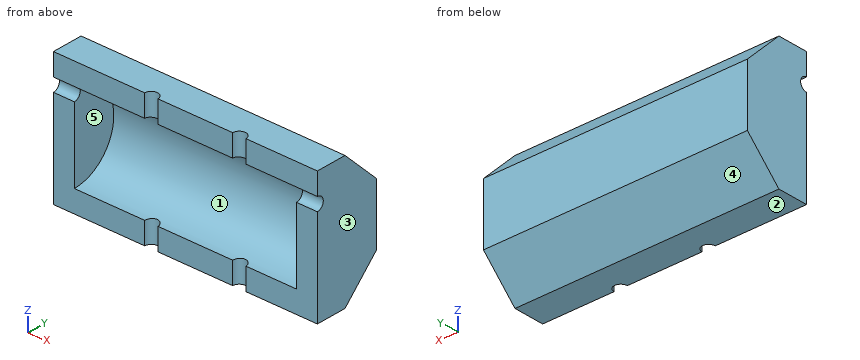
from build123d import *

# Parameters (mm, degrees)
F0_W          = 60
F0_H          = 30
F1_DEPTH      = 15
F3_W          = 50.5
F3_H          = 10
F5_R          = 1.5
F6_DEPTH      = 60.001
F7_R          = 1.5
F8_DEPTH      = 15.001
F8_DEPTH_BACK = 15.001
F9_SIZE       = 8


with BuildPart() as f1:
    # F0 (on Front) → F1 (new body)
    with BuildSketch(Plane.XZ):
        with Locations((30, 0)):
            Rectangle(F0_W, F0_H)
    extrude(amount=-F1_DEPTH)

    # F3 (on Front) → F4 (revolve, cut)
    with BuildSketch(Plane.XZ):
        with Locations((30, 5)):
            Rectangle(F3_W, F3_H)
    revolve(axis=Axis((30, 0, 0), (1, 0, 0)), mode=Mode.SUBTRACT)

    # F5 (on Right) → F6 (cut, through all)
    with BuildSketch(Plane.YZ):
        with Locations((0, 8.5)):
            Circle(F5_R)
    extrude(amount=F6_DEPTH, mode=Mode.SUBTRACT)

    # F7 (on Top) → F8 (cut, two sides)
    with BuildSketch(Plane.XY) as f8_sk:
        with Locations((22.25, 0)):
            Circle(F7_R)
        with Locations((42.25, 0)):
            Circle(F7_R)
    extrude(amount=-F8_DEPTH, mode=Mode.SUBTRACT)
    extrude(f8_sk.sketch, amount=F8_DEPTH_BACK, mode=Mode.SUBTRACT)

    # F9
    f9_edges = [f1.edges().sort_by_distance(p)[0] for p in [
        (30, 15, 15),
        (30, 15, -15),
    ]]
    chamfer(f9_edges, length=F9_SIZE)


solid = f1.part
CAD build for the part. Positions are in the model's coordinates, mm. Face numbers are marked on the shaded views. A direction names the side the tool comes from. Round coordinates to 2 decimals unless told otherwise and drop trailing zeros. Write each loop counter-clockwise with the first axis right and the second up, starting at its lowest first coordinate (ties: lowest second). Pieces come first, ordered by that corner, then holes.
(1) Slice it at C-C, the plane y = 9. Write the cut outline in (x, z), and give its area (3 significant figures).
(2) Slice it at A-A, the plane z = -11.5. Write the cut outline in (x, y).
(3) Slice it at B-B, the plane x = 8. Write the cut outline in (y, z), and give its area (3 significant figures).
(4) Probe line 1 along X through (y, z) = (4.5, -3.5); line 2 along Y through (x, z) = (46, -1.5); line 3 along Z through (x, y) = (22, 9.25). List the from-to ranges inside material, lowest first.
(5) Drop a flat-ended pin along its axis: P1, Ø3, axis at x = 6.5, z = 9.5, coming from the +Y side. Give the stop position or say it passes through.
(6) 3-axis set-ups, long thin cutter, end or side, ignore diameter. For the marked faces 1 and 2: which of +Z, -Z, +X, -X, +Y, -Y reach the whole face in a straight line?
(7) Mould opens along Z. For the marked faces 3, 4 and 5 say: pulls with the +Z half, pulls with the -Z half, needs draft (parallel to the pull), parting line crosses it, or undercut.
From the geometry:
1. outline: (0, -13) - (60, -13) - (60, 13) - (0, 13) - close; hole (4.75, -4.36) - (55.25, -4.36) - (55.25, 4.36) - (4.75, 4.36) - close
1. area: 1,120 mm2
2. outline: (0, 0) - (20.75, 0) arc R1.5 cw to (23.75, 0) - (40.75, 0) arc R1.5 cw to (43.75, 0) - (60, 0) - (60, 10.5) - (0, 10.5) - close
3. outline: (0, -15) - (7, -15) - (15, -7) - (15, 7) - (7, 15) - (0, 15) - (0, 10) arc R10 cw to (0, -10) - close
3. area: 229 mm2
4. line 1: x = 0 to 4.75, 55.25 to 60
4. line 2: y = 9.89 to 15
4. line 3: z = -12.75 to -3.8, 3.8 to 12.75
5. P1: stops at y = 14
6. face 1: -Y
6. face 2: -Z, +X, -X, +Y, -Y
7. face 3: needs draft
7. face 4: pulls with the -Z half
7. face 5: undercut
